Input: dimensioned drawing with shaded views. Units: mm. Origin: part minimum x, y, z. A direction names the side the tool comes from. Give positions to 0.01 mm unless a question says otherwise; leave off trailing zeros. Loops run counter-clockwise (first coordinate to the right, second up) from the corner with the lowest first, then second, coordinate; pieces in that order, holes last.
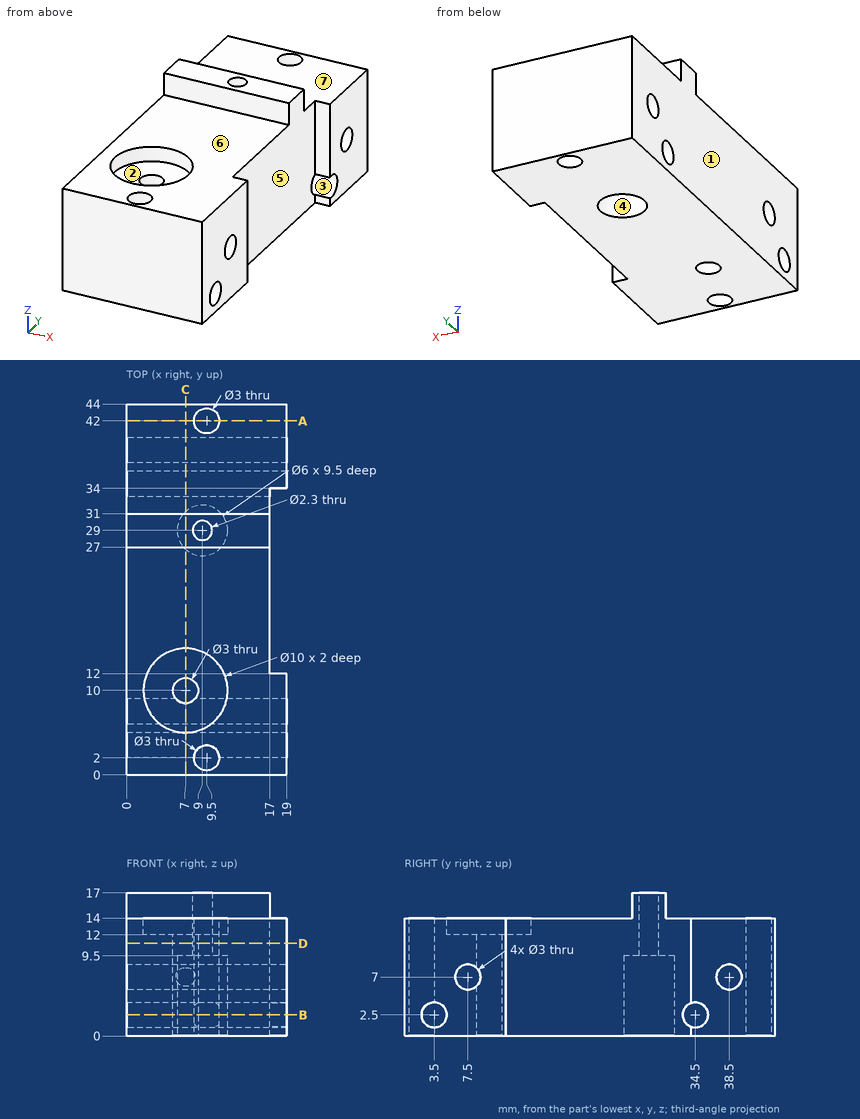
Item 1: Section query C-C on x = 7. Return loops of the section in (y, z), plus the area to 3 significant figures.
Values follow:
outline: (0, 0) - (8.5, 0) - (8.5, 5.88) arc R1.5 cw (long way) to (8.5, 8.12) - (8.5, 12) - (5, 12) - (5, 14) - (0, 14) - close; (11.5, 0) - (26.76, 0) - (26.76, 9.5) - (31.24, 9.5) - (31.24, 0) - (44, 0) - (44, 14) - (31, 14) - (31, 17) - (27, 17) - (27, 14) - (15, 14) - (15, 12) - (11.5, 12) - close; hole circle Ø3 at (3.5, 2.5); hole circle Ø3 at (34.5, 2.5); hole circle Ø3 at (38.5, 7)
area: 502 mm2
Item 2: Draft query along Z for the marked faces 1, 2 and 3. Return one class per face: +Z half, -Z half, draft (parallel to the pull), parting line (faces both ways), or undercut.
Values follow:
face 1: draft
face 2: +Z half
face 3: undercut
Item 3: Section query D-D on z = 11. Return loops of the section in (x, y), plus the area to 3 significant figures.
Values follow:
outline: (0, 0) - (19, 0) - (19, 12) - (17, 12) - (17, 34) - (19, 34) - (19, 44) - (0, 44) - close; hole circle Ø3 at (7, 10); hole circle Ø2.3 at (9, 29); hole circle Ø3 at (9.5, 2); hole circle Ø3 at (9.5, 42)
area: 767 mm2
Item 4: Section query B-B on z = 2.5. Return loops of the section in (x, y), plus the area to 3 significant figures.
Values follow:
outline: (0, 0) - (19, 0) - (19, 2) - (11, 2) arc R1.5 cw to (8, 2) - (0, 2) - close; (0, 5) - (19, 5) - (19, 12) - (17, 12) - (17, 33) - (0, 33) - close; (0, 36) - (19, 36) - (19, 44) - (0, 44) - close; hole circle Ø3 at (7, 10); hole circle Ø6 at (9, 29); hole circle Ø3 at (9.5, 42)
area: 634 mm2
Item 5: Pin query (flat end, axial travel): pin 1 (1.5 mm diameter, centred on x = 7.5, z = 15.5, fed in from +Y); pin 2 (8.5 mm diameter, centred on y = 24, z = 5.5, fed in from +X); pin 3 (5 mm diameter, centred on x = 7, y = 10, fed in from +Z); pin 4 (1.4 mm diameter, centred on x = 9, y = 29, fed in from -Z). Return the tip coordinate at first contact, or that it passes through.
Values follow:
pin 1: stops at y = 31
pin 2: stops at x = 17
pin 3: stops at z = 12
pin 4: passes through
Item 6: Ray query, probe 1 along Z at (x, y) = (10.5, 34.5); probe 2 along Y at (x, z) = (9.5, 6.75); probe 3 along Y at (x, z) = (9, 5.25). Return the intervals inside material, ascending.
Values follow:
probe 1: z = 0 to 1, 4 to 14
probe 2: y = 0 to 0.5, 3.5 to 6.02, 8.98 to 26.04, 31.96 to 37.02, 39.98 to 40.5, 43.5 to 44
probe 3: y = 0 to 0.59, 3.41 to 26, 32 to 40.59, 43.41 to 44
Item 7: Section query A-A on y = 42. Return loops of the section in (x, z).
Values follow:
outline: (0, 0) - (8, 0) - (8, 14) - (0, 14) - close; (11, 0) - (19, 0) - (19, 14) - (11, 14) - close
Item 8: Set-up query: the marked faces 4, 5, 6 and 7. Return all of +Z, -Z, +X, -X, +Y, -Y with unobstructed straight access to the full face (end or side cutting, diameter ignored); none if empty.
Values follow:
face 4: -Z
face 5: +Z, -Z, +X
face 6: +Z, +X, -X, -Y
face 7: +Z, +X, -X, +Y
